Read the model definition and answer for the solid it produces. Units are mm, in the model's axes. A direction names the side the tool comes from. Coordinates: 2 decimals unless noted, no trailing zeros. Loops run counter-clockwise (first coordinate to the right, second up) from the corner with the lowest first, then second, coordinate; pieces in that order, holes last. Notation, with made-up numbers: (20, 75.25) -> (24, 75.25) arc R19 cw to (24, 85.25) -> close; hole circle Ø4 at (40.5, -28.75). An arc over 180 degrees is marked (long way). Answer as CSV lines item,"result".
```python
from build123d import *

# Parameters (mm, degrees)
F0_W     = 11
F0_H     = 112.6
F1_DEPTH = 2
F3_W     = 11
F3_H     = 112.6
F4_DEPTH = 10
F5_R     = 2
F6_R     = 1.5
F7_DEPTH = 25


with BuildPart() as f1:
    # F0 (on Top) → F1 (new body)
    with BuildSketch(Plane.XY):
        Polygon((-31.7652441872, 6.6397131595), (-31.7652441872, 43.2397131595), (-33.7652441872, 43.2397131595), (-33.7652441872, -69.3602868405), (-26.7652441872, -69.3602868405), (-26.7652441872, -49.3602868405), (-32.7652441872, -49.3602868405), (-32.7652441872, -33.3602868405), (-26.7652441872, -33.3602868405), (-26.7652441872, 6.6397131595), align=None)
        with Locations((-39.2652441872, -13.0602868405)):
            Rectangle(F0_W, F0_H)
    extrude(amount=F1_DEPTH)

    # F3 (on offset) → F4 (join)
    with BuildSketch(Plane.XY.offset(2)):
        with Locations((-39.2652441872, -13.0602868405)):
            Rectangle(F3_W, F3_H)
    extrude(amount=F4_DEPTH)

    # F5
    f5_edges = [f1.edges().sort_by_distance(p)[0] for p in [
        (-39.265244, 43.239713, 12),
        (-44.765244, -13.060287, 12),
        (-33.765244, -13.060287, 12),
        (-39.265244, -69.360287, 12),
    ]]
    fillet(f5_edges, radius=F5_R)

    # F6 (on face) → F7 (cut)
    with BuildSketch(Plane.XY.offset(2)):
        with Locations((-29.7272081302, -0.3602868405)):
            Circle(F6_R)
        with Locations((-29.5696301797, -29.3602868405)):
            Circle(F6_R)
        with Locations((-29.3848836171, -63.3602868405)):
            Circle(F6_R)
    extrude(amount=-F7_DEPTH, mode=Mode.SUBTRACT)


solid = f1.part
```
Q1. A cutting plane is placed at B-B, the plane z = 1. Write down the section's boundary in (x, y), and give its area (3 significant figures).
Results:
outline,"(-44.77, -69.36) -> (-26.77, -69.36) -> (-26.77, -49.36) -> (-32.77, -49.36) -> (-32.77, -33.36) -> (-26.77, -33.36) -> (-26.77, 6.64) -> (-31.77, 6.64) -> (-31.77, 43.24) -> (-44.77, 43.24) -> close; hole circle Ø3 at (-29.73, -0.36); hole circle Ø3 at (-29.57, -29.36); hole circle Ø3 at (-29.38, -63.36)"
area,"1,730 mm²"
Q2. Find the intervals of material crossed by probe 1 along Y at (x, z) = (-31.5, 1.5); probe 2 along X at (y, z) = (-42.5, 4.5); probe 3 along X at (y, z) = (-40.5, 10.25), in increasing order. Write a range as [from, to].
Results:
probe 1,"y = [-69.36, -49.36], [-33.36, 6.64]"
probe 2,"x = [-44.77, -33.77]"
probe 3,"x = [-44.75, -33.78]"
Q3. A cutting plane is placed at A-A, the plane y = -19. Write down the section's boundary in (x, z).
Results:
outline,"(-44.77, 0) -> (-26.77, 0) -> (-26.77, 2) -> (-33.77, 2) -> (-33.77, 10) arc R2 ccw to (-35.77, 12) -> (-42.77, 12) arc R2 ccw to (-44.77, 10) -> close"
Q4. For a pull along X with two mould halves and no side action, classify faces 6 (the face through (-31.068, -29.294, 1.014)), 7 (the face through (-38, -12, 0)), 8 (the face through (-26.765, -14, 1)), 9 (the face through (-28.3, 0.1, 1)) as pulls with the +X half, pulls with the -X half, needs draft (parallel to the pull), parting line crosses it, or undercut.
Results:
face 6,"undercut"
face 7,"needs draft"
face 8,"pulls with the +X half"
face 9,"undercut"
Q5. Given pin 1 Ø1 at (x, z) = (-30.5, 1) entering from +Y; pin 2 Ø8 at (x, y) = (-30, 10) entering from +Z; pin 3 Ø4 at (y, z) = (-21, 10) entering from +X, each flat-ended and moving along its own axis, determine where each tip first touches the part or whether it passes through.
Results:
pin 1,"stops at y = 6.64"
pin 2,"stops at z = 10.94"
pin 3,"stops at x = -33.77"
Q6. For faces 1 (the face through (-38, 43.24, 5)), 2 (the face through (-31.765, 25, 1)), 3 (the face through (-44.765, -14, 5)), 4 (the face through (-30, -49.36, 1)), 5 (the face through (-31, -25, 2)), determine the directions among +Z, -Z, +X, -X, +Y, -Y from which every point of the face is accessible in a straight line to the end or side of a thin tool.
Results:
face 1,"+Z, -Z, +X, -X, +Y"
face 2,"+Z, -Z, +X, +Y"
face 3,"+Z, -Z, -X, +Y, -Y"
face 4,"+Z, -Z, +X"
face 5,"+Z, +X, +Y, -Y"
Q7. A cutting plane is placed at C-C, the plane y = 32. Write down the section's boundary in (x, z), and give its area (3 significant figures).
Results:
outline,"(-44.77, 0) -> (-31.77, 0) -> (-31.77, 2) -> (-33.77, 2) -> (-33.77, 10) arc R2 ccw to (-35.77, 12) -> (-42.77, 12) arc R2 ccw to (-44.77, 10) -> close"
area,"134 mm²"
